Check sheet for the modelled part. Datum: model origin and axes. Units: mm. Face numbers are marked on the shaded views. A direction names the side the tool comes from. Give positions to 0.01 mm unless a question says otherwise; leave off trailing zeros. Write each loop counter-clockwise with the first axis right and the second up, starting at its lowest first coordinate (ties: lowest second). Pieces come first, ordered by that corner, then holes. Notation, with made-up numbers: M 25.25,78.25 L 83.25,78.25 A16 cw 83.25,101.25 Z; hole C 16.25,-18.5 d6. An arc over 180 degrees is marked long. Write item = value, one per line. Start each with the question number.
1) Sectioned sample at A-A, the plane z = 28. Record the cut outline in (x, y), then the cut area to 3 significant figures.
2) Scan lines: L1, parallel to X at y = 4.25, z = 55; L2, parallel to Z at x = -51.5, y = 10.5. Record each from-to range of solid material in increasing order.
3) Sectioned sample at B-B, the plane y = 15.5. Record the cut outline in (x, z), then the cut area to 3 significant figures.
4) Gauge pin test, flat ends, axial feed: pin 1 (1.5 mm diameter, centred on x = 9, y = 15, fed in from +Z); pin 2 (9 mm diameter, centred on x = 57, y = 32, fed in from -Z); pin 3 (5 mm diameter, centred on y = 36.5, z = -56, fed in from -X); pin 4 (11 mm diameter, centred on x = -55, z = 55, fed in from +Y). Record the tip position at first contact, or that the pin passes through.
5) Set-up check for the marked faces 1, 2, 3 and 4: record each of +Z, -Z, +X, -X, +Y, -Y from which the full face is reachable in a straight line by a thin tool's end or side.
6) Sectioned sample at C-C, the plane x = -11.5. Record the cut outline in (y, z), then the cut area to 3 significant figures.
7) Sectioned sample at D-D, the plane y = 42. Record the cut outline in (x, z), then the cut area to 3 significant figures.
from build123d import *

# Parameters (mm, degrees)
SKETCH1_R           = 6
BOSS_EXTRUDE2_DEPTH = 12
BOSS_EXTRUDE3_DEPTH = 48
BOSS_EXTRUDE5_DEPTH = 5
BOSS_EXTRUDE6_DEPTH = 10


with BuildPart() as part:
    # Sketch1 → Boss-Extrude2 (new body)
    with BuildSketch(Plane(origin=(0, 0, 0), x_dir=(1, 0, 0), z_dir=(0, 1, 0))):
        with BuildLine():
            Line((-55, 75), (55, 75))
            ThreePointArc((55, 75), (69.142135624, 69.142135624), (75, 55))
            Line((75, 55), (75, -55))
            ThreePointArc((75, -55), (69.142135624, -69.142135624), (55, -75))
            Line((55, -75), (-55, -75))
            ThreePointArc((-55, -75), (-69.142135624, -69.142135624), (-75, -55))
            Line((-75, -55), (-75, 55))
            ThreePointArc((-75, 55), (-69.142135624, 69.142135624), (-55, 75))
        make_face()
        with Locations((-55, 55)):
            Circle(SKETCH1_R, mode=Mode.SUBTRACT)
        with Locations((-55, -55)):
            Circle(SKETCH1_R, mode=Mode.SUBTRACT)
        with Locations((55, -55)):
            Circle(SKETCH1_R, mode=Mode.SUBTRACT)
        with Locations((55, 55)):
            Circle(SKETCH1_R, mode=Mode.SUBTRACT)
    extrude(amount=BOSS_EXTRUDE2_DEPTH)

    # Sketch2 → Boss-Extrude3 (add)
    with BuildSketch(Plane(origin=(0, 12, 0), x_dir=(1, 0, 0), z_dir=(0, 1, 0))):
        with BuildLine():
            Line((-35, 45), (35, 45))
            ThreePointArc((35, 45), (42.071067812, 42.071067812), (45, 35))
            Line((45, 35), (45, -35))
            ThreePointArc((45, -35), (42.071067812, -42.071067812), (35, -45))
            Line((35, -45), (-35, -45))
            ThreePointArc((-35, -45), (-42.071067812, -42.071067812), (-45, -35))
            Line((-45, -35), (-45, 35))
            ThreePointArc((-45, 35), (-42.071067812, 42.071067812), (-35, 45))
        make_face()
    extrude(amount=BOSS_EXTRUDE3_DEPTH)

    # Sketch3 → Boss-Extrude5 (add, symmetric)
    with BuildSketch(Plane(origin=(0, 0, 0), x_dir=(0, 0, -1), z_dir=(1, 0, 0))):
        Polygon((45, 50), (45, 12), (75, 12), align=None)
        Polygon((-45, 12), (-75, 12), (-45, 50), align=None)
    extrude(amount=BOSS_EXTRUDE5_DEPTH, both=True)

    # Sketch6 → Boss-Extrude6 (add)
    with BuildSketch(Plane.XY):
        Polygon((45, 50), (75, 12), (45, 12), align=None)
        Polygon((-45, 50), (-45, 12), (-75, 12), align=None)
    extrude(amount=BOSS_EXTRUDE6_DEPTH)


solid = part.part
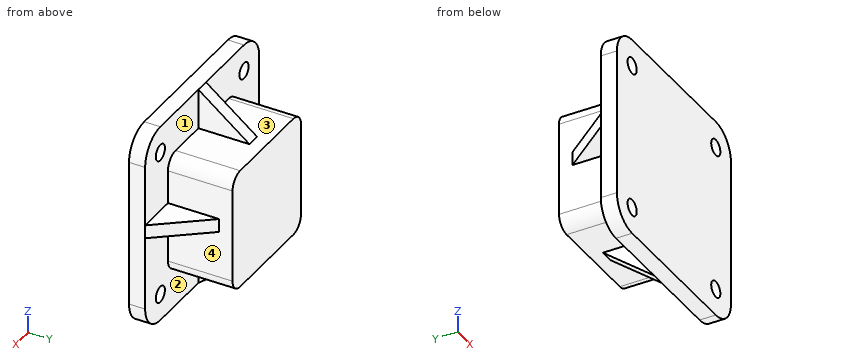
Data:
q1.outline = M -75,0 L 75,0 L 75,12 L 45,12 L 45,60 L -45,60 L -45,12 L -75,12 Z
q1.area = 6,120 mm2
q2.L1 = -75 to -61, -49 to 49, 61 to 75
q2.L2 = -75 to -59.87, -50.13 to 50.13, 59.87 to 75
q3.outline = M -72.24,0 L -45,0 L -45,-35 A10 ccw -35,-45 L -5,-45 L -5,-72.24 L 5,-72.24 L 5,-45 L 35,-45 A10 ccw 45,-35 L 45,0 L 72.24,0 L 72.24,10 L 45,10 L 45,35 A10 ccw 35,45 L 5,45 L 5,72.24 L -5,72.24 L -5,45 L -35,45 A10 ccw -45,35 L -45,10 L -72.24,10 Z
q3.area = 9,100 mm2
q4.pin_1 = 45
q4.pin_2 = 0
q4.pin_3 = -5
q4.pin_4 = through
q5.face_1 = +Z, +X, +Y
q5.face_2 = -Z, +X, +Y
q5.face_3 = +Z, +Y
q5.face_4 = +X, +Y
q6.outline = M 0,-75 L 12,-75 L 12,-45 L 60,-45 L 60,45 L 12,45 L 12,75 L 0,75 Z
q6.area = 6,120 mm2
q7.outline = M -51.32,0 L -45,0 L -45,-35 A10 ccw -35,-45 L -5,-45 L -5,-51.32 L 5,-51.32 L 5,-45 L 35,-45 A10 ccw 45,-35 L 45,0 L 51.32,0 L 51.32,10 L 45,10 L 45,35 A10 ccw 35,45 L 5,45 L 5,51.32 L -5,51.32 L -5,45 L -35,45 A10 ccw -45,35 L -45,10 L -51.32,10 Z
q7.area = 8,270 mm2
